from build123d import *

# Parameters (mm, degrees)
SKETCH_R     = 6
PAD_DEPTH    = 20
SKETCH001_R  = 7
PAD001_DEPTH = 2
CHAMFER_SIZE = 1.5
SKETCH002_R  = 5
PAD002_DEPTH = 2
FILLET_R     = 2


with BuildPart() as part:
    # Sketch → Pad (new body)
    with BuildSketch(Plane.XY):
        Circle(SKETCH_R)
    extrude(amount=PAD_DEPTH)

    # Sketch001 (on Face3 of Pad) → Pad001 (join)
    with BuildSketch(Plane.XY.offset(20)):
        Circle(SKETCH001_R)
    extrude(amount=PAD001_DEPTH)

    # Chamfer
    chamfer_edges = [part.edges().sort_by_distance(p)[0] for p in [
        (-7, 0, 22),
    ]]
    chamfer(chamfer_edges, length=CHAMFER_SIZE)

    # Sketch002 (on Face4 of Chamfer) → Pad002 (join)
    with BuildSketch(Plane.XY.offset(22)):
        Circle(SKETCH002_R)
    extrude(amount=PAD002_DEPTH)

    # Fillet
    fillet_edges = [part.edges().sort_by_distance(p)[0] for p in [
        (-6, 0, 0),
    ]]
    fillet(fillet_edges, radius=FILLET_R)


solid = part.part
Check sheet for the modelled part. Datum: model origin and axes. Units: mm. A direction names the side the tool comes from. Give positions to 0.01 mm unless a question says otherwise; leave off trailing zeros. Write each loop counter-clockwise with the first axis right and the second up, starting at its lowest first coordinate (ties: lowest second). Pieces come first, ordered by that corner, then holes. Notation, with made-up numbers: (-27.75, 68) -> (26.25, 68) arc R21 cw to (26.25, 79) -> close; hole circle Ø10 at (65, 5). An arc over 180 degrees is marked (long way). Use one line per item in the form item = value. Start each with the question number.
1. Access from +Z, -Z, +X, -X, +Y, -Y to the whole of each face (thin tool, end or side, straight path). Record for faces 1 (the cylindrical face through (-6, 0, 11)), 2 (the cylindrical face through (-1.08, -4.88, 22.99)), 3 (the flat face through (0, 0, 24)).
2. Section check A-A (y = 0). Record the cut outline in (x, z).
3. Thickness scan on line 1 along X through (y, z) = (0.25, 4.5); line 2 along Y through (x, z) = (-3, 10); line 3 along Y through (x, z) = (-3.25, 4). Record the ranges inside material, lowest first. Write a range as from..to.
4. Section check C-C (z = 7.5). Record the cut outline in (x, y), and give its area (3 significant figures).
5. Go/stop test with flat-tipped pins: P1, Ø1.5, axis at y = 1.5, z = 21.5, coming from the +X side; P2, Ø4, axis at y = -5, z = 5, coming from the -X side; P3, Ø7, axis at x = 2, y = -1.5, coming from the -Z side; P4, Ø1, axis at x = -3.5, z = 5.5, coming from the +Y side. Record where each tip stops, or that it passes through.
Conclusion:
q1.face_1 = -Z
q1.face_2 = +Z
q1.face_3 = +Z, +X, -X, +Y, -Y
q2.outline = (-7, 20) -> (-6, 20) -> (-6, 2) arc R2 ccw to (-4, 0) -> (4, 0) arc R2 ccw to (6, 2) -> (6, 20) -> (7, 20) -> (7, 20.5) -> (5.5, 22) -> (5, 22) -> (5, 24) -> (-5, 24) -> (-5, 22) -> (-5.5, 22) -> (-7, 20.5) -> close
q3.line_1 = -5.99..5.99
q3.line_2 = -5.2..5.2
q3.line_3 = -5.04..5.04
q4.outline = circle Ø12 at (0, 0)
q4.area = 113 mm²
q5.P1 = 6.6
q5.P2 = -5.2
q5.P3 = 0
q5.P4 = 5.2
